Can you work these out from the model? Positions are in its coordinate system, mm. A direction names the side the tool comes from. Coordinates: 2 decimals unless noted, no trailing zeros. Loops run counter-clockwise (first coordinate to the right, second up) from the corner with the lowest first, then second, coordinate; pieces in that order, holes last.
```python
from build123d import *

# Parameters (mm, degrees)
IZIM1_W                     = 170
IZIM1_H                     = 75
Y_KSEKLIK_EKSTR_ZYON1_DEPTH = 4
KES_EKSTR_ZYON1_DEPTH       = 93.990590922
IZIM3_R                     = 1.6
KES_EKSTR_ZYON2_DEPTH       = 5
IZIM4_R                     = 3.4
KES_EKSTR_ZYON3_DEPTH       = 2.7
RADYUS1_R                   = 4
IZIM5_R                     = 2.55
KES_EKSTR_ZYON4_DEPTH       = 12
IZIM7_R                     = 11
KES_EKSTR_ZYON5_DEPTH       = 4
IZIM6_R                     = 6
KES_EKSTR_ZYON6_DEPTH       = 7.5
Y_KSEKLIK_EKSTR_ZYON2_START = 6
IZIM8_W                     = 42
IZIM8_H                     = 30
IZIM8_R                     = 11
IZIM8_R_2                   = 1.6
Y_KSEKLIK_EKSTR_ZYON2_DEPTH = 6
IZIM9_R                     = 1.6
KES_EKSTR_ZYON7_DEPTH       = 94.248324522
RADYUS2_R                   = 5
IZIM10_R                    = 1.6
KES_EKSTR_ZYON8_DEPTH       = 15
IZIM11_R                    = 3.4
KES_EKSTR_ZYON9_DEPTH       = 3
RADYUS3_R                   = 2
PAH1_SIZE                   = 1


with BuildPart() as part:
    # Çizim1 → Yükseklik-Ekstrüzyon1 (new, symmetric)
    with BuildSketch(Plane.XY):
        Rectangle(IZIM1_W, IZIM1_H)
    extrude(amount=Y_KSEKLIK_EKSTR_ZYON1_DEPTH, both=True)

    # Çizim2 → Kes-Ekstrüzyon1 (cut, through all)
    with BuildSketch(Plane.XY):
        with BuildLine():
            Line((-15.1, -31.85), (15.1, -31.85))
            ThreePointArc((15.1, -31.85), (16.75, -33.5), (15.1, -35.15))
            Line((15.1, -35.15), (-15.1, -35.15))
            ThreePointArc((-15.1, -35.15), (-16.75, -33.5), (-15.1, -31.85))
        make_face()
        with BuildLine():
            Line((-75.1, -31.85), (-44.9, -31.85))
            ThreePointArc((-44.9, -31.85), (-43.25, -33.5), (-44.9, -35.15))
            Line((-44.9, -35.15), (-75.1, -35.15))
            ThreePointArc((-75.1, -35.15), (-76.75, -33.5), (-75.1, -31.85))
        make_face()
        with BuildLine():
            Line((44.9, -31.85), (75.1, -31.85))
            ThreePointArc((75.1, -31.85), (76.75, -33.5), (75.1, -35.15))
            Line((75.1, -35.15), (44.9, -35.15))
            ThreePointArc((44.9, -35.15), (43.25, -33.5), (44.9, -31.85))
        make_face()
    extrude(amount=KES_EKSTR_ZYON1_DEPTH, mode=Mode.SUBTRACT)

    # Çizim3 → Kes-Ekstrüzyon2 (cut, symmetric)
    with BuildSketch(Plane.XY):
        with Locations((30, -33.5)):
            Circle(IZIM3_R)
        with Locations((-30, -33.5)):
            Circle(IZIM3_R)
    extrude(amount=KES_EKSTR_ZYON2_DEPTH, both=True, mode=Mode.SUBTRACT)

    # Çizim4 → Kes-Ekstrüzyon3 (cut)
    with BuildSketch(Plane(origin=(0, 0, -4), x_dir=(-1, 0, 0), z_dir=(0, 0, -1))):
        with Locations((-30, -33.5)):
            Circle(IZIM4_R)
        with Locations((30, -33.5)):
            Circle(IZIM4_R)
    extrude(amount=-KES_EKSTR_ZYON3_DEPTH, mode=Mode.SUBTRACT)

    # Radyus1
    # the kernel refuses this fillet: 4 mm, written as the material it takes off along each edge
    with BuildSketch(Plane(origin=(95, -37.5, -4), x_dir=(0, 1, 0), z_dir=(-1, 0, 0))) as radyus1_piece_1:
        with BuildLine():
            CenterArc((RADYUS1_R, -RADYUS1_R), RADYUS1_R, 90, 90)
            Line((0, -RADYUS1_R), (0, 0))
            Line((0, 0), (RADYUS1_R, 0))
        make_face()
    extrude(amount=190, mode=Mode.SUBTRACT)

    # Çizim5 → Kes-Ekstrüzyon4 (cut)
    with BuildSketch(Plane(origin=(0, 37.5, 0), x_dir=(1, 0, 0), z_dir=(0, 1, 0))):
        with Locations(Location((0, 0, 0), (0, 0, 270))):
            Circle(IZIM5_R)
    extrude(amount=-KES_EKSTR_ZYON4_DEPTH, mode=Mode.SUBTRACT)

    # Çizim7 → Kes-Ekstrüzyon5 (cut)
    with BuildSketch(Plane.XY.offset(4)):
        with Locations((-60.08, -11.5)):
            Circle(IZIM7_R)
        with Locations((60.09, -11.5)):
            Circle(IZIM7_R)
    extrude(amount=-KES_EKSTR_ZYON5_DEPTH, mode=Mode.SUBTRACT)

    # Çizim6 → Kes-Ekstrüzyon6 (cut, symmetric)
    with BuildSketch(Plane.XY):
        with Locations((60.09, -11.5)):
            Circle(IZIM6_R)
        with Locations((-60.08, -11.5)):
            Circle(IZIM6_R)
    extrude(amount=KES_EKSTR_ZYON6_DEPTH, both=True, mode=Mode.SUBTRACT)

    # Çizim8 → Yükseklik-Ekstrüzyon2 (add)
    # profile 1 of 2: a face of its own
    with BuildSketch(Plane.XY.offset(4).offset(Y_KSEKLIK_EKSTR_ZYON2_START)):
        with Locations((-54.08, -11.5)):
            Rectangle(IZIM8_W, IZIM8_H)
        with Locations((-60.08, -11.5)):
            Circle(IZIM8_R, mode=Mode.SUBTRACT)
        with Locations((-39.48, -3)):
            Circle(IZIM8_R_2, mode=Mode.SUBTRACT)
        with Locations((-39.48, -20)):
            Circle(IZIM8_R_2, mode=Mode.SUBTRACT)
    # profile 2 of 2: a face of its own
    with BuildSketch(Plane.XY.offset(4).offset(Y_KSEKLIK_EKSTR_ZYON2_START)):
        with Locations((54.09, -11.5)):
            Rectangle(IZIM8_W, IZIM8_H)
        with Locations((60.09, -11.5)):
            Circle(IZIM8_R, mode=Mode.SUBTRACT)
        with Locations((39.49, -3)):
            Circle(IZIM8_R_2, mode=Mode.SUBTRACT)
        with Locations((39.49, -20)):
            Circle(IZIM8_R_2, mode=Mode.SUBTRACT)
    extrude(amount=-Y_KSEKLIK_EKSTR_ZYON2_DEPTH)

    # Çizim9 → Kes-Ekstrüzyon7 (cut, through all)
    with BuildSketch(Plane.XY.offset(4)):
        with Locations((-39.48, -3)):
            Circle(IZIM9_R)
        with Locations((-39.48, -20)):
            Circle(IZIM9_R)
        with Locations((39.49, -3)):
            Circle(IZIM9_R)
        with Locations((39.49, -20)):
            Circle(IZIM9_R)
    extrude(amount=-KES_EKSTR_ZYON7_DEPTH, mode=Mode.SUBTRACT)

    # Radyus2
    radyus2_edges = [part.edges().sort_by_distance(p)[0] for p in [
        (-75.08, 3.5, 7),
        (-75.08, -26.5, 7),
        (-33.08, -26.5, 7),
        (-33.08, 3.5, 7),
        (33.09, 3.5, 7),
        (33.09, -26.5, 7),
        (75.09, -26.5, 7),
        (75.09, 3.5, 7),
    ]]
    fillet(radyus2_edges, radius=RADYUS2_R)

    # Çizim10 → Kes-Ekstrüzyon8 (cut, symmetric)
    with BuildSketch(Plane.XY.offset(4)):
        with Locations((-74.88, -11.5)):
            Circle(IZIM10_R)
        with Locations((74.89, -11.5)):
            Circle(IZIM10_R)
    extrude(amount=KES_EKSTR_ZYON8_DEPTH, both=True, mode=Mode.SUBTRACT)

    # Çizim11 → Kes-Ekstrüzyon9 (cut)
    with BuildSketch(Plane(origin=(0, 0, -4), x_dir=(-1, 0, 0), z_dir=(0, 0, -1))):
        with Locations((-74.89, -11.5)):
            Circle(IZIM11_R)
        with Locations((-39.49, -3)):
            Circle(IZIM11_R)
        with Locations((-39.49, -20)):
            Circle(IZIM11_R)
        with Locations((39.48, -3)):
            Circle(IZIM11_R)
        with Locations((39.48, -20)):
            Circle(IZIM11_R)
        with Locations((74.88, -11.5)):
            Circle(IZIM11_R)
    extrude(amount=-KES_EKSTR_ZYON9_DEPTH, mode=Mode.SUBTRACT)

    # Radyus3
    # the kernel refuses this fillet: 2 mm, written as the material it takes off along each edge
    with BuildSketch(Plane(origin=(70.09, -1.5, 10), x_dir=(1, 0, 0), z_dir=(0, -1, 0))) as radyus3_piece_1:
        with BuildLine():
            CenterArc((5 - RADYUS3_R, -RADYUS3_R), RADYUS3_R, 0, 90)
            Line((5 - RADYUS3_R, 0), (5, 0))
            Line((5, 0), (5, -RADYUS3_R))
        make_face()
    revolve(axis=Axis((70.09, -1.5, 10), (0, 0, 1)), revolution_arc=90, mode=Mode.SUBTRACT)
    with BuildSketch(Plane(origin=(75.09, -8.087450787, 10), x_dir=(0, 0, -1), z_dir=(0, -1, 0)), Plane(origin=(-75.08, -14.912549213, 10), x_dir=(0, 0, -1), z_dir=(0, 1, 0)), Plane(origin=(-75.08, -21.5, 10), x_dir=(0, 0, -1), z_dir=(0, 1, 0)), Plane(origin=(75.09, -1.5, 10), x_dir=(0, 0, -1), z_dir=(0, -1, 0))) as radyus3_piece_2:
        with BuildLine():
            CenterArc((RADYUS3_R, -RADYUS3_R), RADYUS3_R, 90, 90)
            Line((0, -RADYUS3_R), (0, 0))
            Line((0, 0), (RADYUS3_R, 0))
        make_face()
    extrude(amount=13.412549213, mode=Mode.SUBTRACT)
    with BuildSketch(Plane(origin=(70.09, -21.5, 10), x_dir=(0, -1, 0), z_dir=(-1, 0, 0))) as radyus3_piece_3:
        with BuildLine():
            CenterArc((5 - RADYUS3_R, -RADYUS3_R), RADYUS3_R, 0, 90)
            Line((5 - RADYUS3_R, 0), (5, 0))
            Line((5, 0), (5, -RADYUS3_R))
        make_face()
    revolve(axis=Axis((70.09, -21.5, 10), (0, 0, 1)), revolution_arc=90, mode=Mode.SUBTRACT)
    with BuildSketch(Plane(origin=(70.09, -26.5, 10), x_dir=(0, 0, -1), z_dir=(-1, 0, 0)), Plane(origin=(-38.08, -26.5, 10), x_dir=(0, 0, -1), z_dir=(-1, 0, 0)), Plane(origin=(38.09, 3.5, 10), x_dir=(0, 0, -1), z_dir=(1, 0, 0)), Plane(origin=(-70.08, 3.5, 10), x_dir=(0, 0, -1), z_dir=(1, 0, 0))) as radyus3_piece_4:
        with BuildLine():
            CenterArc((RADYUS3_R, -RADYUS3_R), RADYUS3_R, 90, 90)
            Line((0, -RADYUS3_R), (0, 0))
            Line((0, 0), (RADYUS3_R, 0))
        make_face()
    extrude(amount=32, mode=Mode.SUBTRACT)
    with BuildSketch(Plane(origin=(38.09, -21.5, 10), x_dir=(-1, 0, 0), z_dir=(0, 1, 0))) as radyus3_piece_5:
        with BuildLine():
            CenterArc((5 - RADYUS3_R, -RADYUS3_R), RADYUS3_R, 0, 90)
            Line((5 - RADYUS3_R, 0), (5, 0))
            Line((5, 0), (5, -RADYUS3_R))
        make_face()
    revolve(axis=Axis((38.09, -21.5, 10), (0, 0, 1)), revolution_arc=90, mode=Mode.SUBTRACT)
    with BuildSketch(Plane(origin=(33.09, -21.5, 10), x_dir=(0, 0, -1), z_dir=(0, 1, 0)), Plane(origin=(-33.08, -1.5, 10), x_dir=(0, 0, -1), z_dir=(0, -1, 0))) as radyus3_piece_6:
        with BuildLine():
            CenterArc((RADYUS3_R, -RADYUS3_R), RADYUS3_R, 90, 90)
            Line((0, -RADYUS3_R), (0, 0))
            Line((0, 0), (RADYUS3_R, 0))
        make_face()
    extrude(amount=20, mode=Mode.SUBTRACT)
    with BuildSketch(Plane(origin=(38.09, -1.5, 10), x_dir=(-1, 0, 0), z_dir=(0, -1, 0))) as radyus3_piece_7:
        with BuildLine():
            CenterArc((5 - RADYUS3_R, RADYUS3_R), RADYUS3_R, 270, 90)
            Line((5 - RADYUS3_R, 0), (5, 0))
            Line((5, 0), (5, RADYUS3_R))
        make_face()
    revolve(axis=Axis((38.09, -1.5, 10), (0, 0, -1)), revolution_arc=90, mode=Mode.SUBTRACT)
    with BuildSketch(Plane(origin=(-70.08, -21.5, 10), x_dir=(-1, 0, 0), z_dir=(0, 1, 0))) as radyus3_piece_8:
        with BuildLine():
            CenterArc((5 - RADYUS3_R, -RADYUS3_R), RADYUS3_R, 0, 90)
            Line((5 - RADYUS3_R, 0), (5, 0))
            Line((5, 0), (5, -RADYUS3_R))
        make_face()
    revolve(axis=Axis((-70.08, -21.5, 10), (0, 0, 1)), revolution_arc=90, mode=Mode.SUBTRACT)
    with BuildSketch(Plane(origin=(-38.08, -21.5, 10), x_dir=(0, -1, 0), z_dir=(-1, 0, 0))) as radyus3_piece_9:
        with BuildLine():
            CenterArc((5 - RADYUS3_R, -RADYUS3_R), RADYUS3_R, 0, 90)
            Line((5 - RADYUS3_R, 0), (5, 0))
            Line((5, 0), (5, -RADYUS3_R))
        make_face()
    revolve(axis=Axis((-38.08, -21.5, 10), (0, 0, 1)), revolution_arc=90, mode=Mode.SUBTRACT)
    with BuildSketch(Plane(origin=(-38.08, -1.5, 10), x_dir=(1, 0, 0), z_dir=(0, -1, 0))) as radyus3_piece_10:
        with BuildLine():
            CenterArc((5 - RADYUS3_R, -RADYUS3_R), RADYUS3_R, 0, 90)
            Line((5 - RADYUS3_R, 0), (5, 0))
            Line((5, 0), (5, -RADYUS3_R))
        make_face()
    revolve(axis=Axis((-38.08, -1.5, 10), (0, 0, 1)), revolution_arc=90, mode=Mode.SUBTRACT)
    with BuildSketch(Plane(origin=(-70.08, -1.5, 10), x_dir=(-1, 0, 0), z_dir=(0, -1, 0))) as radyus3_piece_11:
        with BuildLine():
            CenterArc((5 - RADYUS3_R, RADYUS3_R), RADYUS3_R, 270, 90)
            Line((5 - RADYUS3_R, 0), (5, 0))
            Line((5, 0), (5, RADYUS3_R))
        make_face()
    revolve(axis=Axis((-70.08, -1.5, 10), (0, 0, -1)), revolution_arc=90, mode=Mode.SUBTRACT)

    # Pah1
    pah1_edges = [part.edges().sort_by_distance(p)[0] for p in [
        (-71.08, -11.5, 10),
        (49.09, -11.5, 10),
    ]]
    chamfer(pah1_edges, length=PAH1_SIZE)


solid = part.part
```
(1) I want a section at A-A on x = -30. Write out the boundary of the cut face in (y, z).
Check values:
outline: (-37.5, 0) arc R4 ccw to (-36.9, -2.11) - (-36.9, -1.3) - (-35.1, -1.3) - (-35.1, 4) - (-37.5, 4) - close; (-31.9, -1.3) - (-30.1, -1.3) - (-30.1, -4) - (37.5, -4) - (37.5, 4) - (-31.9, 4) - close
(2) I want a section at B-B on x = -11. Write out the boundary of the cut face in (y, z).
Check values:
outline: (-37.5, 0) arc R4 ccw to (-33.5, -4) - (37.5, -4) - (37.5, 4) - (-31.85, 4) - (-31.85, 0) - (-35.15, 0) - (-35.15, 4) - (-37.5, 4) - close
(3) I want a section at D-D on y = -3. State how many separate pieces and enclosed holes the cut face has, then the cut area to 3 significant figures.
Check values:
separate pieces: 3
enclosed holes: 0
area: 1,470 mm2
(4) If we mould it in two halves opening along Y, with no side actions, what happens to faces 6 (the cylindrical face through (-68.81, -18.19, 4.56)), 7 (the cylindrical face through (-73.65, -25, 5.97)), 8 (the flat face through (-54, 3.5, 6))? For each: released by +Y, released by -Y, zero draft, split by the parting line, or undercut.
Check values:
face 6: undercut
face 7: released by -Y
face 8: released by +Y
(5) I'm going to push flat-ended pins straight in: pin 1 (5 mm diameter, centred on x = 49.5, y = 21.5, fed in from +Z); pin 2 (3.5 mm diameter, centred on x = -28.5, y = -33, fed in from -Z); pin 3 (4 mm diameter, centred on x = 0, z = 0.5, fed in from +Y). Where does each tip first touch, or does it pass through?
Check values:
pin 1: stops at z = 4
pin 2: stops at z = -1.3
pin 3: stops at y = 25.5
(6) I want a section at C-C on y = 13. Write out the boundary of the cut face in (x, z).
Check values:
outline: (-85, -4) - (85, -4) - (85, 4) - (-85, 4) - close
(7) Which directions (+Z, -Z, +X, -X, +Y, -Y) give clear straight access to the entire face, cutting with the end or side of a thin tool? Please do faces 1 (the cylindrical face through (41.016, -2.519, 4.577)), 2 (the flat face through (-1, 2, -4)), 3 (the cylindrical face through (-76.75, -33.54, 1.97)), 4 (the flat face through (75.09, -6, 6)), 5 (the flat face through (73, -12, -1)).
Check values:
face 1: +Z, -Z
face 2: -Z, +X, -X, +Y, -Y
face 3: +Z
face 4: +Z, +X, +Y, -Y
face 5: -Z
(8) If I drill on probe 1 along Y at (x, z) = (39.49, 6.25); probe 2 along Y at (x, z) = (73, 0.5); probe 3 along Y at (x, z) = (60.09, 7.25), over which ranges is the centre line in solid material (lowest first)?
Check values:
probe 1: y = -26.5 to -21.6, -18.4 to -4.6, -1.4 to 3.5
probe 2: y = -37.5 to -35.15, -31.85 to 37.5
probe 3: y = -26.5 to -22.5, -0.5 to 3.5
